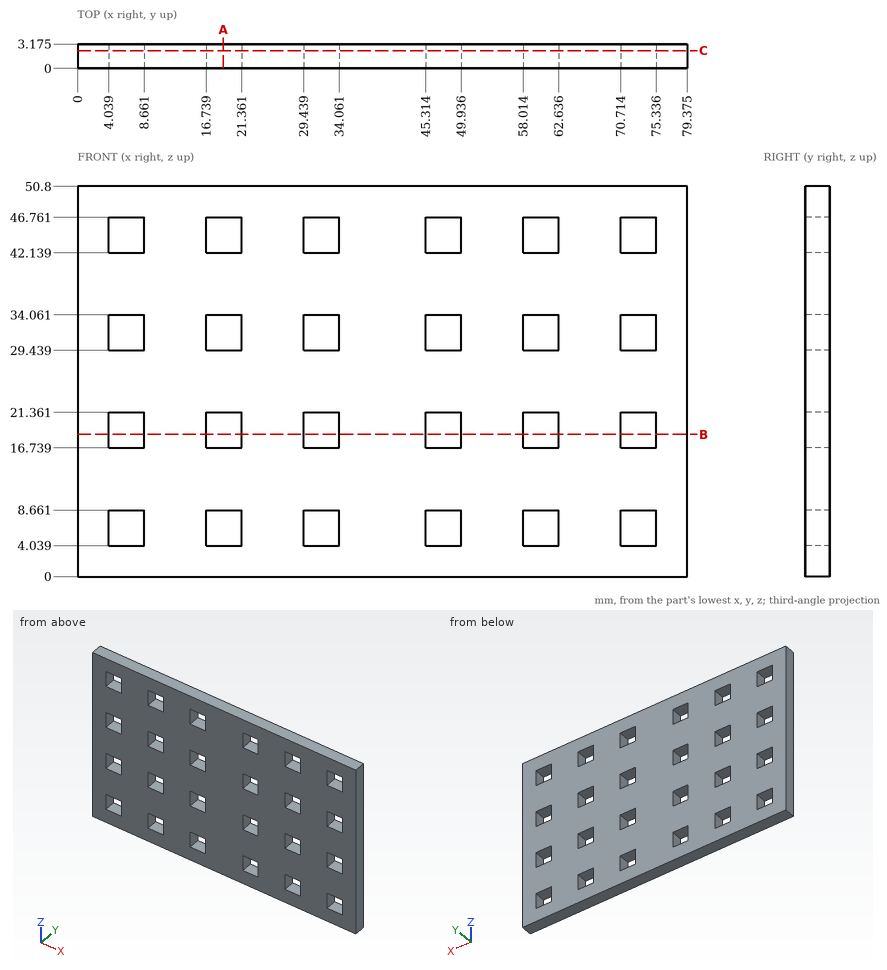
Print and shaded views of the part. All mm, measured from the part's lowest x, y and z. Round coordinates to 2 decimals unless told otherwise and drop trailing zeros. Loops run counter-clockwise (first coordinate to the right, second up) from the corner with the lowest first, then second, coordinate; pieces in that order, holes last. Notation, with made-up numbers: (79.25, 14) -> (98.25, 14) arc R37 cw to (98.25, 51) -> close; hole circle Ø1 at (-32.75, -4). An arc over 180 degrees is marked (long way). Use CSV: the item, a comma, the result in double quotes. Start each with the question number.
1) Cut at A-A, the plane x = 19. Write the cut outline in (y, z) (1 decimal).
2) Cut at B-B, the plane z = 18.5. Write the cut outline in (x, y) (1 decimal), plus the area to 3 significant figures.
3) Wall check: L1, parallel to Z at x = 62, y = 0.6. Give the ranges that are in metal, low to high. Write a range as [from, to].
4) Cut at C-C, the plane y = 2.3. Give the number of separate pieces and of enclosed holes in the cut face, plus the area to 3 significant figures.
Determined:
1,outline,"(0, 0) -> (3.2, 0) -> (3.2, 4) -> (0, 4) -> close; (0, 8.7) -> (3.2, 8.7) -> (3.2, 16.7) -> (0, 16.7) -> close; (0, 21.4) -> (3.2, 21.4) -> (3.2, 29.4) -> (0, 29.4) -> close; (0, 34.1) -> (3.2, 34.1) -> (3.2, 42.1) -> (0, 42.1) -> close; (0, 46.8) -> (3.2, 46.8) -> (3.2, 50.8) -> (0, 50.8) -> close"
2,outline,"(0, 0) -> (4, 0) -> (4, 3.2) -> (0, 3.2) -> close; (8.7, 0) -> (16.7, 0) -> (16.7, 3.2) -> (8.7, 3.2) -> close; (21.4, 0) -> (29.4, 0) -> (29.4, 3.2) -> (21.4, 3.2) -> close; (34.1, 0) -> (45.3, 0) -> (45.3, 3.2) -> (34.1, 3.2) -> close; (49.9, 0) -> (58, 0) -> (58, 3.2) -> (49.9, 3.2) -> close; (62.6, 0) -> (70.7, 0) -> (70.7, 3.2) -> (62.6, 3.2) -> close; (75.3, 0) -> (79.4, 0) -> (79.4, 3.2) -> (75.3, 3.2) -> close"
2,area,"164 mm2"
3,L1,"z = [0, 4.04], [8.66, 16.74], [21.36, 29.44], [34.06, 42.14], [46.76, 50.8]"
4,separate pieces,"1"
4,enclosed holes,"24"
4,area,"3,520 mm2"
